from build123d import *

# Parameters (mm, degrees)
SKETCH1_R           = 4.2
BOSS_EXTRUDE1_DEPTH = 33
SKETCH2_R           = 16
SKETCH2_W           = 40.2
SKETCH2_H           = 40.2
CUT_EXTRUDE1_DEPTH  = 117.571866246
CUT_EXTRUDE2_START  = 10
SKETCH3_R           = 26
CUT_EXTRUDE2_DEPTH  = 107.571866246
SKETCH4_R           = 23.6
CUT_EXTRUDE3_DEPTH  = 3.4
FILLET1_R           = 30
CHAMFER1_SIZE       = 2
CUT_EXTRUDE5_START  = -25
SKETCH5_R           = 6.6
CUT_EXTRUDE5_DEPTH  = 92.571866246
CHAMFER2_SIZE       = 10
BOSS_EXTRUDE2_REACH = 118.572
SKETCH6_R           = 3
SKETCH6_2_R         = 3
CUT_EXTRUDE6_DEPTH  = 119.084715353


with BuildPart() as part:
    # Sketch1 → Boss-Extrude1 (new, symmetric)
    with BuildSketch(Plane(origin=(0, 0, 0), x_dir=(1, 0, 0), z_dir=(0, 1, 0))):
        Polygon((0, 0), (0, -50), (40, -50), (100, -10), (100, 0), align=None)
        with Locations(Location((20, -10, 0), (0, 0, 270))):
            Circle(SKETCH1_R, mode=Mode.SUBTRACT)
        with Locations(Location((20, -40, 0), (0, 0, 270))):
            Circle(SKETCH1_R, mode=Mode.SUBTRACT)
    extrude(amount=BOSS_EXTRUDE1_DEPTH, both=True)

    # Sketch2 → Cut-Extrude1 (cut, through all)
    with BuildSketch(Plane.XY):
        with Locations((70, 0)):
            Circle(SKETCH2_R)
        with Locations((20, 0)):
            Rectangle(SKETCH2_W, SKETCH2_H)
    extrude(amount=CUT_EXTRUDE1_DEPTH, mode=Mode.SUBTRACT)

    # Sketch3 → Cut-Extrude2 (cut, through all)
    with BuildSketch(Plane.XY.offset(CUT_EXTRUDE2_START)):
        with Locations((70, 0)):
            Circle(SKETCH3_R)
    extrude(amount=CUT_EXTRUDE2_DEPTH, mode=Mode.SUBTRACT)

    # Sketch4 → Cut-Extrude3 (cut)
    with BuildSketch(Plane.XY.offset(10)):
        with Locations((70, 0)):
            Circle(SKETCH4_R)
    extrude(amount=-CUT_EXTRUDE3_DEPTH, mode=Mode.SUBTRACT)

    # Fillet1
    fillet1_edges = [part.edges().sort_by_distance(p)[0] for p in [
        (100, 33, 5),
        (100, -33, 5),
    ]]
    fillet(fillet1_edges, radius=FILLET1_R)

    # Chamfer1
    chamfer1_edges = [part.edges().sort_by_distance(p)[0] for p in [
        (40.1, -20.1, 24.966666667),
        (40.1, 20.1, 24.966666667),
    ]]
    chamfer(chamfer1_edges, length=CHAMFER1_SIZE)

    # Sketch5 → Cut-Extrude5 (cut, through all)
    with BuildSketch(Plane(origin=(0, 0, 0), x_dir=(1, 0, 0), z_dir=(0, 1, 0)).offset(CUT_EXTRUDE5_START)):
        with Locations(Location((20, -40, 0), (0, 0, 270))):
            Circle(SKETCH5_R)
        with Locations(Location((20, -10, 0), (0, 0, 270))):
            Circle(SKETCH5_R)
    cut_extrude5 = extrude(amount=-CUT_EXTRUDE5_DEPTH, mode=Mode.SUBTRACT)

    # Mirror1: Cut-Extrude5 across plane
    add(cut_extrude5.mirror(Plane.ZX), mode=Mode.SUBTRACT)

    # Chamfer2
    chamfer2_edges = [part.edges().sort_by_distance(p)[0] for p in [
        (0, -26.55, 50),
        (0, -26.55, 0),
        (0, 26.55, 50),
        (0, 26.55, 0),
    ]]
    chamfer(chamfer2_edges, length=CHAMFER2_SIZE)

    # Boss-Extrude2: up to this plane
    boss_extrude2_end = Plane(origin=(40, 33, 50), z_dir=(-0.5547001962252289, 0, -0.8320502943378438))
    # Sketch6 → Boss-Extrude2 (add, up to the surface)
    with BuildSketch(Plane.XY, mode=Mode.PRIVATE) as boss_extrude2_sk1:
        with BuildLine():
            Line((66.68337521, 27), (73.31662479, 27))
            ThreePointArc((73.31662479, 27), (70, 38), (66.68337521, 27))
        make_face()
        with Locations((70, 32)):
            Circle(SKETCH6_R, mode=Mode.SUBTRACT)
    boss_extrude2_tool1 = split(extrude(boss_extrude2_sk1.sketch, amount=BOSS_EXTRUDE2_REACH, mode=Mode.PRIVATE), bisect_by=boss_extrude2_end, keep=Keep.BOTH, mode=Mode.PRIVATE)
    boss_extrude2 = boss_extrude2_tool1.solids().sort_by_distance((70, 27.162788, 0))[0]
    add(boss_extrude2)

    # Sketch6<2> → Cut-Extrude6 (cut, through all)
    with BuildSketch(Plane.XY):
        with Locations((70, 32)):
            Circle(SKETCH6_2_R)
    cut_extrude6 = extrude(amount=CUT_EXTRUDE6_DEPTH, mode=Mode.SUBTRACT)

    # Mirror2: Boss-Extrude2, Cut-Extrude6 across plane
    add(boss_extrude2.mirror(Plane.ZX))
    add(cut_extrude6.mirror(Plane.ZX), mode=Mode.SUBTRACT)


solid = part.part
Source: CAD feature listing. Evaluate the final solid. Frame: model axes, mm. A direction names the side the tool comes from. Round coordinates to 2 decimals unless told otherwise and drop trailing zeros. Order: outer loops, then holes, each group sorted by start corner. A loop starts at its lowest first (then second) coordinate and runs counter-clockwise, first axis right, second up. Notation, with made-up numbers: (-22, 73) - (23, 73) arc R28 cw to (23, 99) - close; hole circle Ø7 at (-12, -10.75). An arc over 180 degrees is marked (long way). Use a Markdown table: item, result. Add a question column.
1. Section query C-C (y = 13). Return the cut outline in (x, z), then the cut area to 3 significant figures.
2. Section query B-B (x = 37). Return the cut outline in (y, z).
3. Section query D-D (y = 0). Return the cut outline in (x, z), then the cut area to 3 significant figures.
4. Line query: probe 1 along Z at (x, y) = (20, 30); probe 2 along X at (y, z) = (-29.5, 12); probe 3 along Z at (x, y) = (71, -17). Output: solid intervals per line, ascending.
5. Mould query, pull axis Z, two halves, no side actions, for faces 4 (the cylindrical face through (24.164, -22.584, 9.453)), 5 (the flat face through (25, 27, 50)), 6 (the flat face through (32, -33, 25)), 7 (the cylindrical face through (13.557, 28.944, 8.569)). Classes: +Z half, -Z half, draft (parallel to the pull), parting line (faces both ways), or undercut.
6. First-contact query: pin 1 (13.5 mm diameter, centred on x = 20, z = 40, fed in from -Y); pin 2 (9.5 mm diameter, centred on x = 20, z = 10, fed in from -Y); pin 3 (3 mm diameter, centred on x = 36.5, z = 9, fed in from +Y); pin 4 (8 mm diameter, centred on x = 70, y = -32, fed in from -Z). Flat tips, straight axial feed; report the tip coordinate or a pass-through.
7. Section query A-A (x = 70). Return the cut outline in (y, z).
8. Set-up query: faces 1 (the cylindrical face through (13.557, -28.944, 8.569)), 2 (the cylindrical face through (44.025, 1.143, 24.531)), 3 (the flat face through (40.1, 0, 25)). Return all of +Z, -Z, +X, -X, +Y, -Y with unobstructed straight access to the full face (end or side cutting, diameter ignored); none if empty.
Derived:
| question | item | result |
|---|---|---|
| 1 | outline | (40.1, 0) - (60.67, 0) - (60.67, 6.6) - (50.3, 6.6) - (50.3, 10) - (47.48, 10) - (47.48, 45.01) - (40.1, 49.93) - close; (79.33, 0) - (98.28, 0) - (98.28, 11.14) - (92.52, 14.99) - (92.52, 10) - (89.7, 10) - (89.7, 6.6) - (79.33, 6.6) - close |
| 1 | area | 619 mm2 |
| 2 | outline | (-33, 0) - (-20.1, 0) - (-20.1, 50) - (-33, 50) - close; (20.1, 0) - (33, 0) - (33, 50) - (20.1, 50) - close |
| 3 | outline | (40.1, 0) - (54, 0) - (54, 6.6) - (46.4, 6.6) - (46.4, 10) - (44, 10) - (44, 47.33) - (40.1, 49.93) - close; (86, 0) - (100, 0) - (100, 10) - (96, 12.67) - (96, 10) - (93.6, 10) - (93.6, 6.6) - (86, 6.6) - close |
| 3 | area | 383 mm2 |
| 4 | probe 1 | 0 to 3.4, 16.6 to 33.4, 46.6 to 50 |
| 4 | probe 2 | 0 to 13.71, 26.29 to 68.34, 71.66 to 84.06 |
| 4 | probe 3 | 0 to 6.6 |
| 5 | face 4 | undercut |
| 5 | face 5 | +Z half |
| 5 | face 6 | draft |
| 5 | face 7 | undercut |
| 6 | pin 1 | y = -33 |
| 6 | pin 2 | y = -25 |
| 6 | pin 3 | y = 33 |
| 6 | pin 4 | z = 0 |
| 7 | outline | (-38, 0) - (-35, 0) - (-35, 30) - (-38, 30) - close; (-29, 0) - (-16, 0) - (-16, 6.6) - (-23.6, 6.6) - (-23.6, 10) - (-26, 10) - (-26, 30) - (-29, 30) - close; (16, 0) - (29, 0) - (29, 30) - (26, 30) - (26, 10) - (23.6, 10) - (23.6, 6.6) - (16, 6.6) - close; (35, 0) - (38, 0) - (38, 30) - (35, 30) - close |
| 8 | face 1 | -Y |
| 8 | face 2 | +Z |
| 8 | face 3 | +Z, -Z, -X |
